Drawing for the job (mm, zero at the part's lowest x, y, z). A direction names the side the tool comes from. Round coordinates to 2 decimals unless told otherwise and drop trailing zeros. Loops run counter-clockwise (first coordinate to the right, second up) from the corner with the lowest first, then second, coordinate; pieces in that order, holes last.
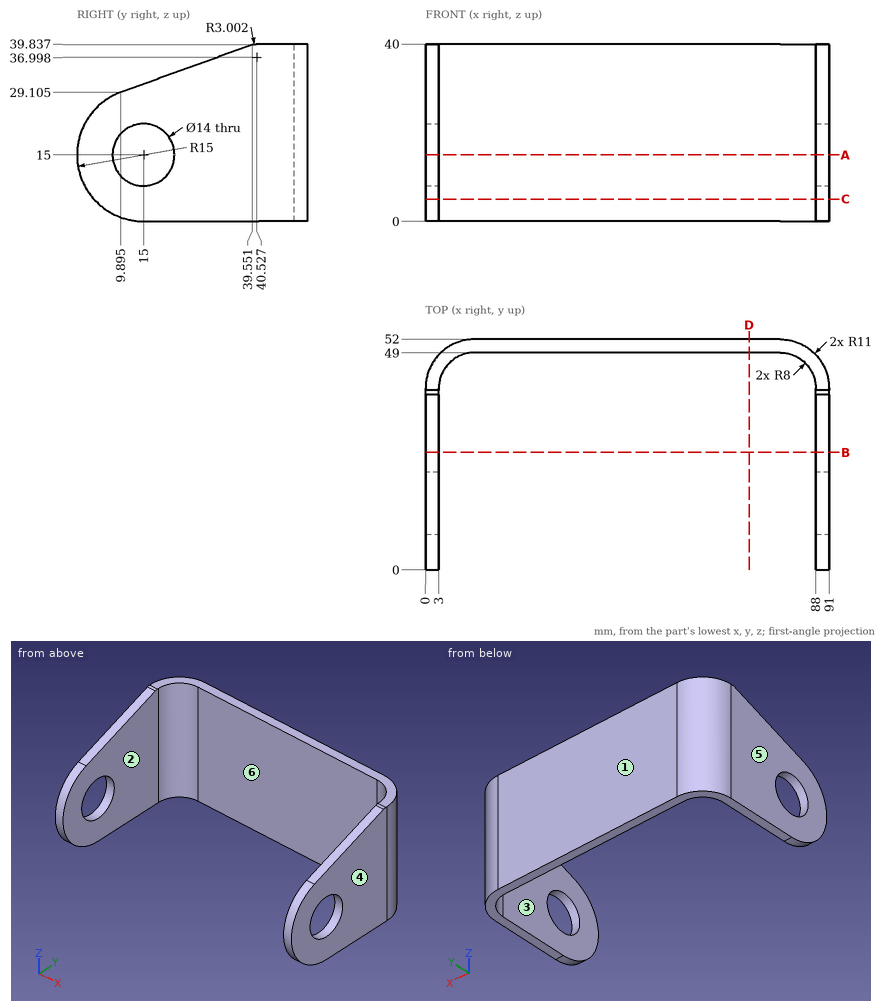
Q1. Slice it at C-C on z = 5. Give the cut face in (x, y).
Q2. Pull direction X, two halves, no side cores. Call the marked faces 3, 4, 5 and 6: pulls with the +X half, pulls with the -X half, needs draft (parallel to the pull), parting line crosses it, or undercut.
Q3. Flat gauge pins, fed straight in: P1, Ø1.5, axis at y = 11.5, z = 31, coming from the -X side; P2, Ø20, axis at x = 35.5, z = 30, coming from the -Y side. Where does each tip first touch, or does it go through?
Q4. Slice it at B-B on y = 26.5. Give the cut face in (x, z) (1 decimal).
Q5. Slice it at A-A on z = 15. Give the cut face in (x, y).
Q6. Slice it at D-D on x = 73. Give the cut face in (y, z), plus the area to 3 significant figures.
Q7. Probe line 1 (X direction, y = 36, z = 11.5); line 2 (Z direction, x = 0.9, y = 15); line 3 (Y direction, x = 23, z = 20). List the from-to ranges inside material, lowest first.
Q8. Tool access for the marked faces 1 and 2: list every direction of +Z, -Z, +X, -X, +Y, -Y with a clear straight run to the whole face (end or side of a thin tool).
Reply:
1. outline: (0, 3.82) - (3, 3.82) - (3, 41) arc R8 cw to (11, 49) - (80, 49) arc R8 cw to (88, 41) - (88, 3.82) - (91, 3.82) - (91, 41) arc R11 ccw to (80, 52) - (11, 52) arc R11 ccw to (0, 41) - close
2. face 3: undercut
2. face 4: pulls with the +X half
2. face 5: pulls with the -X half
2. face 6: undercut
3. P1: passes through
3. P2: stops at y = 49
4. outline: (0, 0) - (3, 0) - (3, 35.1) - (0, 35.1) - close; (88, 0) - (91, 0) - (91, 35.1) - (88, 35.1) - close
5. outline: (0, 0) - (3, 0) - (3, 8) - (0, 8) - close; (0, 22) - (3, 22) - (3, 41) arc R8 cw to (11, 49) - (80, 49) arc R8 cw to (88, 41) - (88, 22) - (91, 22) - (91, 41) arc R11 ccw to (80, 52) - (11, 52) arc R11 ccw to (0, 41) - close; (88, 0) - (91, 0) - (91, 8) - (88, 8) - close
6. outline: (49, 0) - (52, 0) - (52, 40) - (49, 40) - close
6. area: 120 mm2
7. line 1: x = 0 to 3, 88 to 91
7. line 2: z = 0 to 8, 22 to 30.95
7. line 3: y = 49 to 52
8. face 1: +Z, -Z, +X, -X, +Y
8. face 2: +Z, -Z, -Y
